Build history of the part. All positions in model axes, mm. Round coordinates to 2 decimals unless told otherwise and drop trailing zeros. Loops run counter-clockwise (first coordinate to the right, second up) from the corner with the lowest first, then second, coordinate; pieces in that order, holes last. Notation, with made-up numbers: (-16.75, -22.75) - (22.25, -22.75) arc R33 cw to (22.25, 5.25) - close; hole circle Ø11 at (89.25, -31.75). An arc over 180 degrees is marked (long way). Use one line per item in the form item = value. Start each with the question number.
Q1. Drill centre lines: line 1 (Y direction, x = 10, z = 5.5); line 2 (Y direction, x = -7.5, z = 0.5). Where is each one in solid material? Low to high.
Q2. Saw through at B-B (z = 5). Give the cut face in (x, y).
Q3. Pin check, flat tip, straight feed: pin 1 (3 mm diameter, centred on x = 10, y = 10, fed in from +Z). Stop position of the tip, or through.
Q4. Saw through at A-A (y = 10). Give the cut face in (x, z).
Q5. Saw through at D-D (z = 7.5). Give the cut face in (x, y).
```python
from build123d import *

# Parameters (mm, degrees)
SKETCH_1_W         = 30
SKETCH_1_H         = 30
EXTRUDE_1_DEPTH    = 8
HOLE_WIZARD_M4_1_D = 3.3
CHAMFER_1_SIZE     = 3
FILLET_1_R         = 2
CHAMFER_2_SIZE     = 1


with BuildPart() as part:
    # ｽｹｯﾁ1 → ﾎﾞｽ - 押し出し1 (new body)
    with BuildSketch(Plane.XY):
        Rectangle(SKETCH_1_W, SKETCH_1_H)
    extrude(amount=EXTRUDE_1_DEPTH)

    # M4 すきま穴1 (through all)
    with Locations(Plane.XY.offset(8)):
        with Locations((-10, 10), (-10, -10), (10, -10), (10, 10)):
            Hole(HOLE_WIZARD_M4_1_D / 2)

    # 面取り1
    chamfer_1_edges = [part.edges().sort_by_distance(p)[0] for p in [
        (-15, 15, 4),
        (15, 15, 4),
        (15, -15, 4),
        (-15, -15, 4),
    ]]
    chamfer(chamfer_1_edges, length=CHAMFER_1_SIZE)

    # ﾌｨﾚｯﾄ1
    fillet_1_edges = [part.edges().sort_by_distance(p)[0] for p in [
        (-12, 15, 4),
        (12, 15, 4),
        (15, -12, 4),
        (15, 12, 4),
        (-15, -12, 4),
        (-15, 12, 4),
        (-12, -15, 4),
        (12, -15, 4),
    ]]
    fillet(fillet_1_edges, radius=FILLET_1_R)

    # 面取り2
    chamfer_2_edges = [part.edges().sort_by_distance(p)[0] for p in [
        (15, 0, 0),
        (15, 0, 8),
        (13.5, 13.5, 8),
        (0, 15, 8),
        (-13.5, 13.5, 8),
        (-15, 0, 8),
        (-13.5, -13.5, 8),
        (0, -15, 8),
        (13.5, -13.5, 8),
        (11.93693974, -14.847759065, 8),
        (14.847759065, -11.93693974, 8),
        (-11.93693974, -14.847759065, 8),
        (-14.847759065, -11.93693974, 8),
        (-14.847759065, 11.93693974, 8),
        (-11.93693974, 14.847759065, 8),
        (11.93693974, 14.847759065, 8),
        (14.847759065, 11.93693974, 8),
        (13.5, 13.5, 0),
        (0, 15, 0),
        (13.5, -13.5, 0),
        (0, -15, 0),
        (-13.5, -13.5, 0),
        (-15, 0, 0),
        (-13.5, 13.5, 0),
        (11.93693974, -14.847759065, 0),
        (14.847759065, -11.93693974, 0),
        (-11.93693974, -14.847759065, 0),
        (-14.847759065, -11.93693974, 0),
        (-14.847759065, 11.93693974, 0),
        (-11.93693974, 14.847759065, 0),
        (11.93693974, 14.847759065, 0),
        (14.847759065, 11.93693974, 0),
    ]]
    chamfer(chamfer_2_edges, length=CHAMFER_2_SIZE)


solid = part.part
```
Report:
q1.line_1 = -15 to -11.65, -8.35 to 8.35, 11.65 to 15
q1.line_2 = -14.5 to 14.5
q2.outline = (-15, -11.17) arc R2 ccw to (-14.41, -12.59) - (-12.59, -14.41) arc R2 ccw to (-11.17, -15) - (11.17, -15) arc R2 ccw to (12.59, -14.41) - (14.41, -12.59) arc R2 ccw to (15, -11.17) - (15, 11.17) arc R2 ccw to (14.41, 12.59) - (12.59, 14.41) arc R2 ccw to (11.17, 15) - (-11.17, 15) arc R2 ccw to (-12.59, 14.41) - (-14.41, 12.59) arc R2 ccw to (-15, 11.17) - close; hole circle Ø3.3 at (-10, -10); hole circle Ø3.3 at (-10, 10); hole circle Ø3.3 at (10, -10); hole circle Ø3.3 at (10, 10)
q3.pin_1 = through
q4.outline = (-15, 1) - (-14, 0) - (-11.65, 0) - (-11.65, 8) - (-14, 8) - (-15, 7) - close; (-8.35, 0) - (8.35, 0) - (8.35, 8) - (-8.35, 8) - close; (11.65, 0) - (14, 0) - (15, 1) - (15, 7) - (14, 8) - (11.65, 8) - close
q5.outline = (-14.5, -11.17) arc R1.5 ccw to (-14.06, -12.23) - (-12.23, -14.06) arc R1.5 ccw to (-11.17, -14.5) - (11.17, -14.5) arc R1.5 ccw to (12.23, -14.06) - (14.06, -12.23) arc R1.5 ccw to (14.5, -11.17) - (14.5, 11.17) arc R1.5 ccw to (14.06, 12.23) - (12.23, 14.06) arc R1.5 ccw to (11.17, 14.5) - (-11.17, 14.5) arc R1.5 ccw to (-12.23, 14.06) - (-14.06, 12.23) arc R1.5 ccw to (-14.5, 11.17) - close; hole circle Ø3.3 at (-10, -10); hole circle Ø3.3 at (-10, 10); hole circle Ø3.3 at (10, -10); hole circle Ø3.3 at (10, 10)
